```python
from build123d import *

# Parameters (mm, degrees)
F0_W           = 59.7585067153
F0_H           = 44.6528843604
F0_R           = 5.5279344662
F1_DEPTH       = 25.4
F2_D           = 5
F2_DEPTH       = 15.0876
F2_CSINK_D     = 7.62
F2_CSINK_ANGLE = 90
F2_TIP         = 1.5021515476


with BuildPart() as f1:
    # F0 (on Front) → F1 (new body)
    with BuildSketch(Plane.XZ):
        with Locations((-55.9406019747, 29.6302598435)):
            Rectangle(F0_W, F0_H)
        with Locations((-61.0864721239, 33.8631533086)):
            Circle(F0_R, mode=Mode.SUBTRACT)
        with Locations((-61.0864721239, 33.8631533086)):
            Circle(F0_R)
    extrude(amount=-F1_DEPTH)

    # F2
    with Locations(Plane.XZ):
        with Locations((-61.0864721239, 33.8631533086)):
            CounterSinkHole(F2_D / 2, F2_CSINK_D / 2, depth=F2_DEPTH, counter_sink_angle=F2_CSINK_ANGLE)
            with Locations((0, 0, -(F2_DEPTH + F2_TIP / 2))):  # 118° drill point
                Cone(0, F2_D / 2, F2_TIP, mode=Mode.SUBTRACT)


solid = f1.part
```
For this review, take the finished solid that the model builds, in its own axes (mm). Round coordinates to 2 decimals unless told otherwise and drop trailing zeros. Write each question's results on one line, items separated by ' | '.
Item 1: For pin 1 (1.5 mm diameter, centred on x = -52, z = 29.5, fed in from -Y), flat-tipped, find the tip position at first contact; note if it passes through.
Calculated:
pin 1: stops at y = 0
Item 2: Draft analysis for pull direction Z (two halves, no side actions). For faces 1 (the face through (-56, 13, 51.957)), 2 (the face through (-63.396, 8.295, 32.906)), 3 (the face through (-85.82, 13, 29)), state which applies: pulls with the +Z half, pulls with the -Z half, needs draft (parallel to the pull), parting line crosses it, or undercut.
Calculated:
face 1: pulls with the +Z half | face 2: undercut | face 3: needs draft
Item 3: To check wall thickness, follow line 1 along Z through (x, y) = (-59.5, 13.5). State the ranges of the line that lie inside material, in increasing order. Write a range as from..to.
Calculated:
line 1: z = 7.3..31.93, 35.8..51.96
